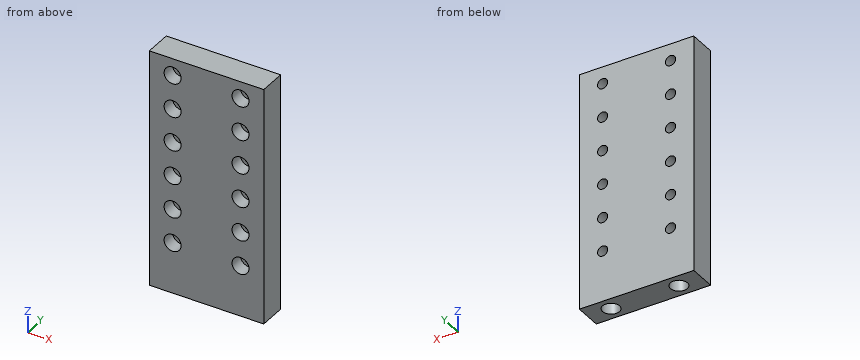
from build123d import *

# Parameters (mm, degrees)
SKETCH_1_W             = 33.7
SKETCH_1_H             = 8
EXTRUDE_1_DEPTH        = 70
SKETCH_2_R             = 2.5
CUT_EXTRUDE_1_DEPTH    = 10
SKETCH_3_R             = 2.5
CUT_EXTRUDE_2_DEPTH    = 4
SKETCH_4_R             = 1.5
CUT_EXTRUDE_3_DEPTH    = 4
PATTERN_LINEAR_1_COUNT = 6
PATTERN_LINEAR_1_PITCH = 10


with BuildPart() as part:
    # 草图1 → 凸台-拉伸1 (new body)
    with BuildSketch(Plane.XY):
        Rectangle(SKETCH_1_W, SKETCH_1_H)
    extrude(amount=EXTRUDE_1_DEPTH)

    # 草图2 → 切除-拉伸1 (cut)
    with BuildSketch(Plane(origin=(0, 0, 0), x_dir=(-1, 0, 0), z_dir=(0, 0, -1))):
        with Locations((10, 0)):
            Circle(SKETCH_2_R)
        with Locations((-10, 0)):
            Circle(SKETCH_2_R)
    extrude(amount=-CUT_EXTRUDE_1_DEPTH, mode=Mode.SUBTRACT)

    # 草图3 → 切除-拉伸2 (cut)
    with BuildSketch(Plane.XZ.offset(4)):
        with Locations(Location((-10, 15, 0), (0, 0, 270))):
            Circle(SKETCH_3_R)
        with Locations(Location((10, 15, 0), (0, 0, 270))):
            Circle(SKETCH_3_R)
    cut_extrude_2 = extrude(amount=-CUT_EXTRUDE_2_DEPTH, mode=Mode.SUBTRACT)

    # 草图4 → 切除-拉伸3 (cut)
    with BuildSketch(Plane(origin=(0, 0, 0), x_dir=(-1, 0, 0), z_dir=(0, -1, 0))):
        with Locations(Location((10, -15, 0), (0, 0, 90))):
            Circle(SKETCH_4_R)
        with Locations(Location((-10, -15, 0), (0, 0, 90))):
            Circle(SKETCH_4_R)
    cut_extrude_3 = extrude(amount=-CUT_EXTRUDE_3_DEPTH, mode=Mode.SUBTRACT)

    # 阵列(线性)1: 切除-拉伸2, 切除-拉伸3 ×6
    with Locations(*[(0, 0, i * PATTERN_LINEAR_1_PITCH) for i in range(1, PATTERN_LINEAR_1_COUNT)]):
        add(cut_extrude_2, mode=Mode.SUBTRACT)
        add(cut_extrude_3, mode=Mode.SUBTRACT)


solid = part.part
Here's how the part is built. I have some questions about the finished solid (model axes, mm). Coordinates: 2 decimals unless noted, no trailing zeros. Loops run counter-clockwise (first coordinate to the right, second up) from the corner with the lowest first, then second, coordinate; pieces in that order, holes last. Notation, with made-up numbers: (85.5, 13.5) -> (99.5, 13.5) arc R13 cw to (99.5, 36.5) -> close; hole circle Ø1 at (88, 65). An arc over 180 degrees is marked (long way). Use one line per item in the form item = value. Start each with the question number.
(1) Will this pin go through, and if not, where does the flat tip stop? pin 1 (2.5 mm diameter, centred on x = 11, z = 54.5, fed in from -Y).
(2) If we section it at B-B (x = 10): Give the number of separate pieces and of enclosed holes in the cut face, then the cut area to 3 significant figures.
(3) If we section it at D-D (z = 65.5): Please give me the cut outline in (x, y).
(4) If we section it at C-C (z = 6.5): Please give me the cut outline in (x, y), then the cut area to 3 significant figures.
(5) If we section it at A-A (z = 45): Please give me the cut outline in (x, y), then the cut area to 3 significant figures.
(6) Please list where these lines run through material, in increasing order: line 1 along X through (y, z) = (-1.45, 25); line 2 along X through (y, z) = (-1, 13); line 3 along Y through (x, z) = (-12, 55.5).
Verdict:
q1.pin_1 = 0
q2.separate_pieces = 7
q2.enclosed_holes = 0
q2.area = 318 mm²
q3.outline = (-16.85, -4) -> (-12.45, -4) -> (-12.45, 0) -> (-11.41, 0) -> (-11.41, 4) -> (-16.85, 4) -> close; (-8.59, 0) -> (-7.55, 0) -> (-7.55, -4) -> (7.55, -4) -> (7.55, 0) -> (8.59, 0) -> (8.59, 4) -> (-8.59, 4) -> close; (11.41, 0) -> (12.45, 0) -> (12.45, -4) -> (16.85, -4) -> (16.85, 4) -> (11.41, 4) -> close
q4.outline = (-16.85, -4) -> (16.85, -4) -> (16.85, 4) -> (-16.85, 4) -> close; hole circle Ø5 at (-10, 0); hole circle Ø5 at (10, 0)
q4.area = 230 mm²
q5.outline = (-16.85, -4) -> (-12.5, -4) -> (-12.5, 0) -> (-11.5, 0) -> (-11.5, 4) -> (-16.85, 4) -> close; (-8.5, 0) -> (-7.5, 0) -> (-7.5, -4) -> (7.5, -4) -> (7.5, 0) -> (8.5, 0) -> (8.5, 4) -> (-8.5, 4) -> close; (11.5, 0) -> (12.5, 0) -> (12.5, -4) -> (16.85, -4) -> (16.85, 4) -> (11.5, 4) -> close
q5.area = 206 mm²
q6.line_1 = -16.85 to -12.5, -7.5 to 7.5, 12.5 to 16.85
q6.line_2 = -16.85 to -11.5, -8.5 to 8.5, 11.5 to 16.85
q6.line_3 = 0 to 4
